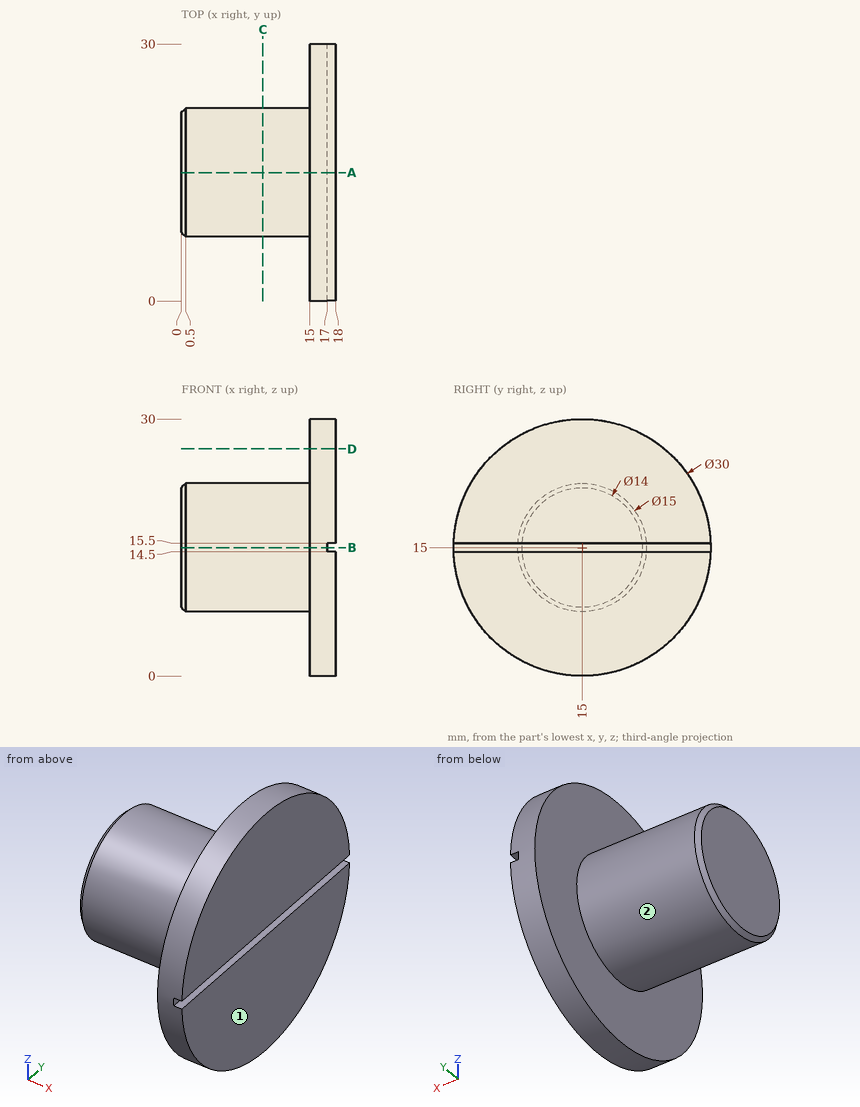
Answer from the drawing. Dimensions are ordinates in mm from the lowest x, y and z of the part. A direction names the side the tool comes from. Round coordinates to 2 decimals unless told otherwise and drop trailing zeros. Write each loop counter-clockwise with the first axis right and the second up, starting at its lowest first coordinate (ties: lowest second). Pieces come first, ordered by that corner, then holes.
1. Given pin 1 Ø5 at (y, z) = (14, 4.5) entering from -X; pin 2 Ø0.8 at (x, y) = (17.5, 19.5) entering from -Z; pin 3 Ø1 at (x, z) = (12.5, 8.5) entering from +Y, each flat-ended and moving along its own axis, determine where each tip first touches the part or whether it passes through.
2. Which of the six approach directions +Z, -Z, +X, -X, +Y, -Y give full straight-line access (tool end or side, diameter ignored) to the marked faces 1 and 2?
3. The part is cut by section A-A, the plane y = 15. Determine the outline of the cut face in (x, z), then the cut area to 3 significant figures.
4. The part is cut by section D-D, the plane z = 26.5. Determine the outline of the cut face in (x, y), then the cut area to 3 significant figures.
5. The part is cut by section C-C, the plane x = 9.5. Determine the outline of the cut face in (y, z).
6. Straight lines are drawn through the part: L1, parallel to X at y = 9.75, z = 3; L2, parallel to Y at x = 4.5, z = 17.75; L3, parallel to Y at x = 1.75, z = 13.5. For each, find the intervals that lie inside material, in ascending order.
7. The part is cut by section B-B, the plane z = 15. Determine the outline of the cut face in (x, y).
Values:
1. pin 1: stops at x = 15
1. pin 2: stops at z = 0.57
1. pin 3: stops at y = 19.5
2. face 1: +Z, -Z, +X, +Y, -Y
2. face 2: -X
3. outline: (0, 8) - (0.5, 7.5) - (15, 7.5) - (15, 0) - (18, 0) - (18, 14.5) - (17, 14.5) - (17, 15.5) - (18, 15.5) - (18, 30) - (15, 30) - (15, 22.5) - (0.5, 22.5) - (0, 22) - close
3. area: 314 mm2
4. outline: (15, 5.37) - (18, 5.37) - (18, 24.63) - (15, 24.63) - close
4. area: 57.8 mm2
5. outline: circle Ø15 at (15, 15)
6. L1: x = 15 to 18
6. L2: y = 8.02 to 21.98
6. L3: y = 7.65 to 22.35
7. outline: (0, 8) - (0.5, 7.5) - (15, 7.5) - (15, 0) - (17, 0) - (17, 30) - (15, 30) - (15, 22.5) - (0.5, 22.5) - (0, 22) - close
